from build123d import *

# Parameters (mm, degrees)
F0_W      = 12.3
F0_H      = 12.1
F1_DEPTH  = 1.76
F2_W      = 8
F2_H      = 0.45
F2_H_2    = 7.8699186992
F3_DEPTH  = 8.3
F5_DEPTH  = 10.151
F7_DEPTH  = 12.101
F9_DEPTH  = 12.301
F11_DEPTH = 10.061


with BuildPart() as f1:
    # F0 (on Top) → F1 (new body)
    with BuildSketch(Plane.XY):
        with Locations((-6.15, 6.05)):
            Rectangle(F0_W, F0_H)
    extrude(amount=F1_DEPTH)

    # F2 (on face) → F3 (join)
    with BuildSketch(Plane.XY.offset(1.76)):
        with Locations((-6.15, 10.2099593496)):
            Rectangle(F2_W, F2_H)
        with Locations((-6.15, 6.05)):
            Rectangle(F2_W, F2_H_2)
        with Locations((-6.15, 1.8900406504)):
            Rectangle(F2_W, F2_H)
    extrude(amount=F3_DEPTH)

    # F4 (on face) → F5 (cut, through all)
    with BuildSketch(Plane(origin=(-10.15, 0, 0), x_dir=(0, -1, 0), z_dir=(-1, 0, 0))):
        Polygon((-10.4349593496, 3.26), (-9.05, 10.06), (-10.4349593496, 10.06), align=None)
        Polygon((-4.55, 10.06), (-7.55, 10.06), (-6.3, 1.76), (-5.8, 1.76), align=None)
        Polygon((-1.6650406504, 10.06), (-3.05, 10.06), (-1.6650406504, 3.26), align=None)
        Polygon((-10.4349593496, 1.76), (-9.6849593496, 1.76), (-9.6849593496, 2.76), (-10.4349593496, 3.26), align=None)
        Polygon((-2.4150406504, 2.76), (-2.4150406504, 1.76), (-1.6650406504, 1.76), (-1.6650406504, 3.26), align=None)
    extrude(amount=-F5_DEPTH, mode=Mode.SUBTRACT)

    # F6 (on Front) → F7 (cut, through all)
    with BuildSketch(Plane.XZ):
        Polygon((-10.15, 10.06), (-10.15, 3.26), (-9.15, 10.06), align=None)
        Polygon((-3.15, 10.06), (-2.15, 3.26), (-2.15, 10.06), align=None)
    extrude(amount=-F7_DEPTH, mode=Mode.SUBTRACT)

    # F8 (on face) → F9 (cut, through all)
    with BuildSketch(Plane(origin=(-12.3, 0, 0), x_dir=(0, -1, 0), z_dir=(-1, 0, 0))):
        with BuildLine():
            ThreePointArc((-6.8, 0), (-6.05, -0.75), (-5.3, 0))
            Line((-5.3, 0), (-6.8, 0))
        make_face()
        with BuildLine():
            Line((-6.8, 0), (-5.3, 0))
            ThreePointArc((-5.3, 0), (-6.05, 0.75), (-6.8, 0))
        make_face()
    extrude(amount=-F9_DEPTH, mode=Mode.SUBTRACT)

    # F10 (on face) → F11 (cut, through all)
    with BuildSketch(Plane(origin=(0, 0, 0), x_dir=(1, 0, 0), z_dir=(0, 0, -1))):
        with BuildLine():
            ThreePointArc((-7.7311388301, -5.3), (-6.5343872054, -7.7572628609), (-4.4, -6.05))
            ThreePointArc((-4.4, -6.05), (-4.4427371391, -5.6656127946), (-4.5688611699, -5.3))
            Line((-4.5688611699, -5.3), (-7.7311388301, -5.3))
        make_face()
        with BuildLine():
            Line((-7.7311388301, -5.3), (-4.5688611699, -5.3))
            ThreePointArc((-4.5688611699, -5.3), (-6.15, -4.3), (-7.7311388301, -5.3))
        make_face()
    extrude(amount=-F11_DEPTH, mode=Mode.SUBTRACT)


solid = f1.part
Read the model definition and answer for the solid it produces. Units are mm, in the model's axes. A direction names the side the tool comes from. Round coordinates to 2 decimals unless told otherwise and drop trailing zeros. Write each loop counter-clockwise with the first axis right and the second up, starting at its lowest first coordinate (ties: lowest second). Pieces come first, ordered by that corner, then holes.
1. Determine the mould class of faces 1 (the face through (-6, 3, 0)), 2 (the face through (-4, 6, 1.76)), 3 (the face through (-6, 9.685, 2)), 4 (the face through (-10.15, 4, 2)) for opening direction Z: pulls with the +Z half, pulls with the -Z half, needs draft (parallel to the pull), parting line crosses it, or undercut.
2. Straight lines are drawn through the part: L1, parallel to Y at x = -9, z = 4; L2, parallel to X at y = 4.5, z = 2; L3, parallel to Z at x = -1, y = 10.5. For each, find the intervals that lie inside material, in ascending order.
3. The part is cut by section B-B, the plane z = 4.5. Determine the outline of the cut face in (x, y).
4. Which of the six approach directions +Z, -Z, +X, -X, +Y, -Y give full straight-line access (tool end or side, diameter ignored) to faces 5 (the face through (-10.15, 8, 2)), 6 (the face through (-8.622, 5.184, 5.852)), 7 (the face through (-6, 8, 10.06)), 8 (the face through (-2.15, 4, 2)), 9 (the face through (-6, 2.415, 2))?
5. Given pin 1 Ø0.5 at (y, z) = (5, 2.5) entering from +X; pin 2 Ø3 at (y, z) = (2, 8.5) entering from -X; pin 3 Ø1.2 at (y, z) = (3.5, 3) entering from -X, each flat-ended and moving along its own axis, determine where each tip first touches the part or whether it passes through.
6. The part is cut by section C-C, the plane x = -3.5. Determine the outline of the cut face in (y, z), then the cut area to 3 significant figures.
7. The part is cut by section D-D, the plane z = 8. Determine the outline of the cut face in (x, y), then the cut area to 3 significant figures.
8. The part is cut by section A-A, the plane x = -6.15. Determine the outline of the cut face in (y, z), then the cut area to 3 significant figures.
Values:
1. face 1: pulls with the -Z half
1. face 2: undercut
1. face 3: undercut
1. face 4: needs draft
2. L1: y = 1.82 to 5.46, 6.64 to 10.28
2. L2: x = -10.15 to -6.96, -5.34 to -2.15
2. L3: z = 0 to 1.76
3. outline: (-9.97, 1.92) - (-2.33, 1.92) - (-2.33, 5.39) - (-4.53, 5.39) arc R1.75 cw to (-7.77, 5.39) - (-9.97, 5.39) - close; (-9.97, 6.71) - (-7.77, 6.71) arc R1.75 cw to (-4.53, 6.71) - (-2.33, 6.71) - (-2.33, 10.18) - (-9.97, 10.18) - close
4. face 5: +Z, -X, +Y, -Y
4. face 6: +Z, +X, -X
4. face 7: +Z, +X, -X, +Y, -Y
4. face 8: +Z, +X, +Y, -Y
4. face 9: +X, -X, -Y
5. pin 1: stops at x = -2.15
5. pin 2: stops at x = -9.59
5. pin 3: stops at x = -10.15
6. outline: (0, 0) - (5.3, 0) arc R0.75 cw to (6.8, 0) - (12.1, 0) - (12.1, 1.76) - (9.68, 1.76) - (9.68, 2.76) - (10.43, 3.26) - (9.05, 10.06) - (7.55, 10.06) - (6.3, 1.76) - (5.8, 1.76) - (4.55, 10.06) - (3.05, 10.06) - (1.67, 3.26) - (2.42, 2.76) - (2.42, 1.76) - (0, 1.76) - close
6. area: 67.4 mm2
7. outline: (-9.45, 2.63) - (-2.85, 2.63) - (-2.85, 4.86) - (-4.87, 4.86) arc R1.75 cw to (-7.43, 4.86) - (-9.45, 4.86) - close; (-9.45, 7.24) - (-7.43, 7.24) arc R1.75 cw to (-4.87, 7.24) - (-2.85, 7.24) - (-2.85, 9.47) - (-9.45, 9.47) - close
7. area: 27.5 mm2
8. outline: (0, 0) - (4.3, 0) - (4.3, 10.06) - (3.05, 10.06) - (1.67, 3.26) - (2.42, 2.76) - (2.42, 1.76) - (0, 1.76) - close; (7.8, 0) - (12.1, 0) - (12.1, 1.76) - (9.68, 1.76) - (9.68, 2.76) - (10.43, 3.26) - (9.05, 10.06) - (7.8, 10.06) - close
8. area: 47.6 mm2
